Can you work these out from the model? Positions are in its coordinate system, mm. Face numbers are marked on the shaded views. A direction names the side the tool comes from. Give positions to 0.01 mm unless a question says otherwise; leave off trailing zeros. Order: outer loops, then holes, each group sorted by start corner. A loop starts at its lowest first (then second) coordinate and runs counter-clockwise, first axis right, second up. Notation, with made-up numbers: (-37.75, 41.25) -> (-1.75, 41.25) arc R16 ccw to (-1.75, 47.25) -> close; hole circle Ø4 at (19.5, -19.5). An arc over 180 degrees is marked (long way). Answer as a JSON object with one key per item and string values.
```python
from build123d import *

# Parameters (mm, degrees)
F0_R     = 15
F1_DEPTH = 50
F3_DEPTH = 10
F2_R     = 17.5
F4_DEPTH = 40
F7_DEPTH = 35
F8_DEPTH = 30


with BuildPart() as f1:
    # F0 (on Right) → F1 (new body)
    with BuildSketch(Plane.YZ):
        Circle(F0_R)
    extrude(amount=F1_DEPTH)

    # F2 (on face) → F3 (join)
    with BuildSketch(Plane.YZ.offset(50)):
        with BuildLine():
            ThreePointArc((-13.9053721633, 5.625), (-5.6082968512, -21.5770023354), (17.5, -5))
            ThreePointArc((17.5, -5), (16.5770023354, 0.6082968512), (13.9053721633, 5.625))
            ThreePointArc((13.9053721633, 5.625), (14.7238001625, 2.8652589369), (15, 0))
            ThreePointArc((15, 0), (-2.8652589369, -14.7238001625), (-13.9053721633, 5.625))
        make_face()
        with BuildLine():
            ThreePointArc((15, 0), (14.7238001625, 2.8652589369), (13.9053721633, 5.625))
            ThreePointArc((13.9053721633, 5.625), (0, 12.5), (-13.9053721633, 5.625))
            ThreePointArc((-13.9053721633, 5.625), (-2.8652589369, -14.7238001625), (15, 0))
        make_face()
    extrude(amount=-F3_DEPTH)

    # F2 (on face) → F4 (join)
    with BuildSketch(Plane.YZ.offset(50)):
        with Locations((0, -5)):
            Circle(F2_R)
    extrude(amount=F4_DEPTH)

    # F6 (on face) → F7 (cut)
    with BuildSketch(Plane.YZ.offset(90)):
        with BuildLine():
            ThreePointArc((12.7377392029, 7), (0, 12.5), (-12.7377392029, 7))
            Line((-12.7377392029, 7), (-5, 7))
            Line((-5, 7), (-5, 0))
            ThreePointArc((-5, 0), (0, -5), (5, 0))
            Line((5, 0), (5, 7))
            Line((5, 7), (12.7377392029, 7))
        make_face()
    extrude(amount=-F7_DEPTH, mode=Mode.SUBTRACT)

    # F6 (on face) → F8 (cut)
    with BuildSketch(Plane.YZ.offset(90)):
        with BuildLine():
            Line((-5, 7), (-12.7377392029, 7))
            ThreePointArc((-12.7377392029, 7), (-16.8994794889, -9.5450624864), (-5, -21.7705098312))
            Line((-5, -21.7705098312), (-5, 0))
            Line((-5, 0), (-5, 7))
        make_face()
    extrude(amount=-F8_DEPTH, mode=Mode.SUBTRACT)


solid = f1.part
```
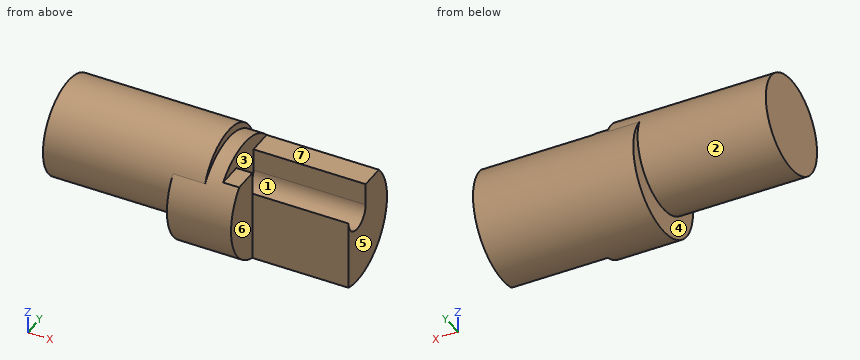
1. If we section it at B-B on x = 79.5: Please give me the cut outline in (y, z).
Worked answers:
{"outline": "(-5, -21.77) arc R17.5 ccw to (12.74, 7) -> (5, 7) -> (5, 0) arc R5 cw to (-5, 0) -> close"}
2. If we section it at D-D on y = 9.5: Please give me the cut outline in (x, z).
Worked answers:
{"outline": "(0, -11.61) -> (40, -11.61) -> (40, -19.7) -> (90, -19.7) -> (90, 7) -> (55, 7) -> (55, 9.7) -> (50, 9.7) -> (50, 11.61) -> (0, 11.61) -> close"}
3. Will these pins go through, and if not, where does the flat tip stop? pin 1 Ø4 at (x, z) = (33.5, 8.5) entering from -Y; pin 2 Ø9 at (y, z) = (-3, 6) entering from +X; pin 3 Ø1.5 at (y, z) = (-1.5, 5) entering from -X; pin 4 Ø10 at (x, z) = (60, -14) entering from +Y.
Worked answers:
{"pin 1": "y = -13.52", "pin 2": "x = 60", "pin 3": "x = 0", "pin 4": "y = 17.04"}
4. Please list where these lines run through material, in increasing order: L1, parallel to Z at x = 43.5, y = 0; L2, parallel to X at y = 12, z = 8; L3, parallel to X at y = 3.5, z = 3.5.
Worked answers:
{"L1": "-22.5 to 15", "L2": "0 to 50", "L3": "0 to 55"}
5. For the marked faces 5, 6 and 7, which set-ups out of +Z, -Z, +X, -X, +Y, -Y let a thin tool reach every point of the face, with its end or its side?
Worked answers:
{"face 5": "+Z, -Z, +X, +Y, -Y", "face 6": "+Z, -Z, +X, -Y", "face 7": "+Z, +X, +Y, -Y"}
6. If we section it at A-A on y = 0: Please give me the cut outline in (x, z).
Worked answers:
{"outline": "(0, -15) -> (40, -15) -> (40, -22.5) -> (90, -22.5) -> (90, -5) -> (55, -5) -> (55, 12.5) -> (50, 12.5) -> (50, 15) -> (0, 15) -> close"}
7. If we mould it in two halves opening along Y, with no side actions, what happens to the marked faces 1, 2, 3 and 4? For each: +Y half, -Y half, draft (parallel to the pull), parting line (faces both ways), or undercut.
Worked answers:
{"face 1": "undercut", "face 2": "parting line", "face 3": "undercut", "face 4": "draft"}
8. If we section it at C-C on z = -17: Please give me the cut outline in (x, y), then the cut area to 3 significant figures.
Worked answers:
{"outline": "(40, -12.74) -> (60, -12.74) -> (60, -5) -> (90, -5) -> (90, 12.74) -> (40, 12.74) -> close", "area": "1,040 mm²"}
